Solid Edge part; units mm, degrees
sketch "Sketch1" plane through (0, 0, 0) normal (0, -1, 0) x (1, 0, 0)
  arc A0 (-5, 0) -> (5, 0) centre (0, 0) ccw
  line L0 (5, 5) -> (5, 0)
  line L1 (-5, 5) -> (5, 5)
  line L2 (-5, 0) -> (-5, 5)
  dimension "D1" = 5
extrude "Extrusionsausprägung_2" add sketch "Sketch1" against normal blind 74
sketch "Sketch2" plane through (0, 74, 0) normal (0, 1, 0) x (1, 0, 0)
  circle A0 centre (0, 0) radius 1.875
extrude "Cutout1" cut sketch "Sketch2" against normal up to next
chamfer "Fase_1" distance 0.5 angle 60 2 edges at (-1.875, 74, 0) (0, 0, 1.875) measured on face at (-3.2333, 0, 3.4333) measured on face at (-3.2333, 74, 3.4333)
properties material "Nylon, allgemein"
Check sheet for the modelled part. Datum: model origin and axes. Units: mm. Coordinates: 2 decimals unless noted, no trailing zeros. Loops run counter-clockwise (first coordinate to the right, second up) from the corner with the lowest first, then second, coordinate; pieces in that order, holes last.
1) Gauge pin test, flat ends, axial feed: pin 1 (1.5 mm diameter, centred on y = 33.5, z = -2.5, fed in from +X); pin 2 (1 mm diameter, centred on y = 31, z = -3, fed in from +X). Record the tip position at first contact, or that the pin passes through.
2) Material ranges on probe 1 along Z at (x, y) = (0, 38) (3 decimals); probe 2 along Z at (x, y) = (1.5, 28) (3 decimals), recorded low to high.
3) Release check for a two-part mould opening along Z. For faces 1 (the face through (0, 36, 5)), 2 (the face through (-1.873, 37.506, -0.082)), 3 (the face through (0, 36, -5)), 4 (the face through (1.2, 0, 2.3)) record: released by +Z, released by -Z, zero draft, split by the parting line, or undercut.
4) Sectioned sample at C-C (z = -3). Record the boundary of the cut face in (x, y).
5) Sectioned sample at D-D (x = -3). Record the boundary of the cut face in (y, z), and give its area (3 significant figures).
6) Sectioned sample at B-B (y = 11). Record the boundary of the cut face in (x, z) (3 decimals), and give its area (3 significant figures).
7) Sectioned sample at A-A (x = 0). Record the boundary of the cut face in (y, z) (3 decimals).
Check sheet entries:
1. pin 1: stops at x = 4.68
1. pin 2: stops at x = 4.33
2. probe 1: z = -5 to -1.875, 1.875 to 5
2. probe 2: z = -4.77 to -1.125, 1.125 to 5
3. face 1: released by +Z
3. face 2: undercut
3. face 3: released by -Z
3. face 4: zero draft
4. outline: (-4, 0) - (4, 0) - (4, 74) - (-4, 74) - close
5. outline: (0, -4) - (74, -4) - (74, 5) - (0, 5) - close
5. area: 666 mm2
6. outline: (-5, 0) arc R5 ccw to (5, 0) - (5, 5) - (-5, 5) - close; hole circle Ø3.75 at (0, 0)
6. area: 78.2 mm2
7. outline: (0, -5) - (74, -5) - (74, -2.375) - (73.134, -1.875) - (0.866, -1.875) - (0, -2.375) - close; (0, 2.375) - (0.866, 1.875) - (73.134, 1.875) - (74, 2.375) - (74, 5) - (0, 5) - close
